Can you work these out from the model? Positions are in its coordinate system, mm. A direction names the side the tool comes from. Coordinates: 2 decimals unless noted, no trailing zeros. Loops run counter-clockwise (first coordinate to the right, second up) from the corner with the lowest first, then second, coordinate; pieces in that order, holes last.
```python
from build123d import *

# Parameters (mm, degrees)
SKETCH_1_W      = 30
SKETCH_1_H      = 15
EXTRUDE_1_DEPTH = 1
EXTRUDE_2_DEPTH = 4


with BuildPart() as part:
    # Sketch 1 → Extrude 1 (new body)
    with BuildSketch(Plane.XY):
        Rectangle(SKETCH_1_W, SKETCH_1_H)
    extrude(amount=EXTRUDE_1_DEPTH)

    # Sketch 1_3 → Extrude 2 (add)
    with BuildSketch(Plane.XY):
        Polygon((15, 7.5), (-15, 7.5), (-9.217262909, 14.5), (9.217262909, 14.5), align=None)
        with BuildLine():
            ThreePointArc((5, 9), (7, 11), (5, 13))
            Line((5, 13), (-5, 13))
            ThreePointArc((-5, 13), (-7, 11), (-5, 9))
            Line((-5, 9), (5, 9))
        make_face(mode=Mode.SUBTRACT)
    extrude(amount=EXTRUDE_2_DEPTH)


solid = part.part
```
Item 1: I'm going to push flat-ended pins straight in: P1, Ø2, axis at x = 1, z = 2.5, coming from the -Y side; P2, Ø1, axis at y = 4, z = 2, coming from the -X side; P3, Ø1.5, axis at x = -5.5, y = 0, coming from the +Z side; P4, Ø1.5, axis at x = -6, y = 0, coming from the -Z side. Where does each tip first touch, or does it pass through?
Results are:
P1: stops at y = 7.5
P2: passes through
P3: stops at z = 1
P4: stops at z = 0
Item 2: Suppose I cut it at A-A, the plane x = 3.5. Please give me the cut outline in (y, z), plus the area to 3 significant figures.
Results are:
outline: (-7.5, 0) - (9, 0) - (9, 4) - (7.5, 4) - (7.5, 1) - (-7.5, 1) - close; (13, 0) - (14.5, 0) - (14.5, 4) - (13, 4) - close
area: 27.0 mm2
Item 3: Suppose I cut it at D-D, the plane x = -8. Please give me the cut outline in (y, z).
Results are:
outline: (-7.5, 0) - (14.5, 0) - (14.5, 4) - (7.5, 4) - (7.5, 1) - (-7.5, 1) - close
Item 4: On a 3-axis mill with a long thin cutter (end or side, diameter ignored), from which of +Z, -Z, +X, -X, +Y, -Y can I reach the whole of each face in a straight line? I mean faces 4 (the face through (12.068, 11.049, 1.972)), 5 (the face through (-7, 11, 2)), 6 (the face through (0, 7.5, 2)). Say none if no direction works.
Results are:
face 4: +Z, -Z, +X, +Y
face 5: +Z, -Z
face 6: +Z, +X, -X, -Y
Item 5: I need wall thicknesses on line 1 along Y through (x, z) = (0.5, 3.2); line 2 along Y through (x, z) = (-0.25, 0.5); line 3 along Z through (x, y) = (10.5, 0.5). Which ranges of each line are inside material? Lowest first, please.
Results are:
line 1: y = 7.5 to 9, 13 to 14.5
line 2: y = -7.5 to 9, 13 to 14.5
line 3: z = 0 to 1
Item 6: Suppose I cut it at C-C, the plane y = 11. Please give me the cut outline in (x, z), plus the area to 3 significant figures.
Results are:
outline: (-12.11, 0) - (-7, 0) - (-7, 4) - (-12.11, 4) - close; (7, 0) - (12.11, 0) - (12.11, 4) - (7, 4) - close
area: 40.9 mm2
Item 7: We'd pull the mould along X, two halves only. Please class faces 1 (the face through (-12.15, 10.95, 1.97)), 2 (the face through (-0.2, -7.5, 0.5)), 3 (the face through (0, 13, 2)): +X half, -X half, draft (parallel to the pull), parting line (faces both ways), or undercut.
Results are:
face 1: -X half
face 2: draft
face 3: undercut
Item 8: Suppose I cut it at B-B, the plane z = 2.8. Please give me the cut outline in (x, y).
Results are:
outline: (-15, 7.5) - (15, 7.5) - (9.22, 14.5) - (-9.22, 14.5) - close; hole (-5, 9) - (5, 9) arc R2 ccw to (5, 13) - (-5, 13) arc R2 ccw to start
